Geometry check sheet. Reference: the model listing, model coordinates, mm. A direction names the side the tool comes from. Round coordinates to 2 decimals unless told otherwise and drop trailing zeros. Write each loop counter-clockwise with the first axis right and the second up, starting at its lowest first coordinate (ties: lowest second). Pieces come first, ordered by that corner, then holes. Notation, with made-up numbers: M 20,-26 L 25,-26 A35 cw 25,10 Z; hole C -22.5,72.5 d5. An arc over 180 degrees is marked long. Answer as CSV lines item,"result". Start each with the question number.
```python
from build123d import *

# Parameters (mm, degrees)
F0_W      = 30
F0_H      = 20
F1_DEPTH  = 100
F2_W      = 80
F2_H      = 80
F3_DEPTH  = 60
F4_W      = 10
F4_H      = 10
F5_DEPTH  = 40
F7_DEPTH  = 30
F9_DEPTH  = 30
F10_W     = 10
F10_H     = 10
F11_DEPTH = 30
F12_W     = 40
F12_H     = 85
F13_DEPTH = 25
F15_W     = 33.7672308087
F15_H     = 41.9678427279
F16_DEPTH = 85
F14_W     = 30
F14_H     = 70
F17_DEPTH = 10
F18_W     = 33.7672308087
F18_H     = 41.9678427279
F19_DEPTH = 15
F20_W     = 40.303826414
F20_H     = 30.5195645853
F21_DEPTH = 10
F22_W     = 47.274120152
F22_H     = 29.6948088799
F23_DEPTH = 100
F25_DEPTH = 30
F27_DEPTH = 5


with BuildPart() as f1:
    # F0 (on Top) → F1 (new body)
    with BuildSketch(Plane.XY):
        Polygon((-33.6863899055, 46.2346871942), (-73.6863899055, 46.2346871942), (-73.6863899055, 16.2346871942), (-73.6863899055, -3.7106291857), (-33.6863899055, -3.7653128058), (-33.6863899055, 16.2346871942), align=None)
        Polygon((106.3136100945, 46.2346871942), (-33.6863899055, 46.2346871942), (-33.6863899055, 16.2346871942), (-3.6863899055, 16.2346871942), (106.3136100945, 16.2346871942), align=None)
        with Locations((-18.6863899055, 6.2346871942)):
            Rectangle(F0_W, F0_H)
    extrude(amount=F1_DEPTH)

    # F2 (on face) → F3 (cut)
    with BuildSketch(Plane(origin=(0, 46.2346871942, 0), x_dir=(-1, 0, 0), z_dir=(0, 1, 0))):
        Polygon((-106.3136100945, 100), (-106.3136100945, 0), (-6.3136100945, 100), align=None)
        with Locations((33.6863899055, 40)):
            Rectangle(F2_W, F2_H)
    extrude(amount=-F3_DEPTH, mode=Mode.SUBTRACT)

    # F4 (on face) → F5 (cut)
    with BuildSketch(Plane(origin=(0, 46.2346871942, 0), x_dir=(-1, 0, 0), z_dir=(0, 1, 0))):
        with Locations((-11.3136100945, 95)):
            Rectangle(F4_W, F4_H)
        with Locations((-101.3136100945, 5)):
            Rectangle(F4_W, F4_H)
        with Locations((-91.3136100945, 15)):
            Rectangle(F4_W, F4_H)
        with Locations((-81.3136100945, 25)):
            Rectangle(F4_W, F4_H)
        with Locations((-71.3136100945, 35)):
            Rectangle(F4_W, F4_H)
        with Locations((-61.3136100945, 45)):
            Rectangle(F4_W, F4_H)
        with Locations((-51.3136100945, 55)):
            Rectangle(F4_W, F4_H)
        with Locations((-41.3136100945, 65)):
            Rectangle(F4_W, F4_H)
        with Locations((-31.3136100945, 75)):
            Rectangle(F4_W, F4_H)
        with Locations((-21.3136100945, 85)):
            Rectangle(F4_W, F4_H)
    extrude(amount=-F5_DEPTH, mode=Mode.SUBTRACT)

    # F6 (on face) → F7 (cut)
    with BuildSketch(Plane.YZ.offset(-3.6863899055)):
        Polygon((16.2346871942, 80), (-3.7653128058, 100), (-3.7653128058, 80), align=None)
    extrude(amount=-F7_DEPTH, mode=Mode.SUBTRACT)

    # F8 (on face) → F9 (join)
    with BuildSketch(Plane.YZ.offset(-3.6863899055)):
        Polygon((-3.7653128058, 120), (-3.7653128058, 100), (16.2346871942, 100), align=None)
    extrude(amount=-F9_DEPTH)

    # F10 (on face) → F11 (cut)
    with BuildSketch(Plane.YZ.offset(-3.6863899055)):
        with Locations((11.2346871942, 105)):
            Rectangle(F10_W, F10_H)
        with Locations((1.2346871942, 115)):
            Rectangle(F10_W, F10_H)
    extrude(amount=-F11_DEPTH, mode=Mode.SUBTRACT)

    # F12 (on face) → F13 (join, symmetric)
    with BuildSketch(Plane(origin=(-0.0052104714, -3.8113580263, 0), x_dir=(0.9999990655, -0.0013670892, 0), z_dir=(-0.0013670892, -0.9999990655, 0))):
        with Locations((-53.6812109081, 142.5)):
            Rectangle(F12_W, F12_H)
    extrude(amount=F13_DEPTH, both=True)

    # F15 (on face) → F16 (cut)
    with BuildSketch(Plane.XY.offset(185)):
        with Locations((-53.6770410836, -4.4620987028)):
            Rectangle(F15_W, F15_H)
    extrude(amount=-F16_DEPTH, mode=Mode.SUBTRACT)

    # F14 (on face) → F17 (cut)
    with BuildSketch(Plane(origin=(0.0289667593, 21.188618612, 0), x_dir=(-0.9999990655, 0.0013670892, 0), z_dir=(0.0013670892, 0.9999990655, 0))):
        with Locations((53.6812109081, 135)):
            Rectangle(F14_W, F14_H)
    extrude(amount=-F17_DEPTH, mode=Mode.SUBTRACT)

    # F18 (on face) → F19 (join)
    with BuildSketch(Plane.XY.offset(185)):
        with Locations((-53.6770410836, -4.4620987028)):
            Rectangle(F18_W, F18_H)
    extrude(amount=-F19_DEPTH)

    # F20 (on face) → F21 (join)
    with BuildSketch(Plane(origin=(0, 0, 100), x_dir=(1, 0, 0), z_dir=(0, 0, -1))):
        with Locations((-53.5686165504, 13.4508235825)):
            Rectangle(F20_W, F20_H)
    extrude(amount=F21_DEPTH)

    # F22 (on face) → F23 (cut)
    with BuildSketch(Plane(origin=(0, 0, 90), x_dir=(1, 0, 0), z_dir=(0, 0, -1))):
        with Locations((-54.1594289243, 18.5580336256)):
            Rectangle(F22_W, F22_H)
    extrude(amount=-F23_DEPTH, mode=Mode.SUBTRACT)

    # F24 (on face) → F25 (cut)
    with BuildSketch(Plane(origin=(0, 46.2346871942, 0), x_dir=(-1, 0, 0), z_dir=(0, 1, 0))):
        Polygon((-72.805352509, 0), (-6.3136100945, 0), (-6.3136100945, 80), align=None)
    extrude(amount=-F25_DEPTH, mode=Mode.SUBTRACT)

    # F26 (on face) → F27 (join)
    with BuildSketch(Plane.XZ.offset(-16.2346871942)):
        Polygon((-3.6863899055, 80), (-3.6863899055, 0), (72.805352509, 0), (6.3136100945, 80), align=None)
    extrude(amount=-F27_DEPTH)


solid = f1.part
```
1) Section check C-C, the plane y = 26.5. Record the cut outline in (x, z).
2) Scan lines: line 1 (X direction, y = 0, z = 142); line 2 (Z direction, x = -60.5, y = 17); line 3 (X direction, y = 18, z = 19). Record each from-to range of solid material in increasing order. Write a range as from..to.
3) Access from +Z, -Z, +X, -X, +Y, -Y to the whole of each face (thin tool, end or side, straight path). Record for faces 1 (the flat face through (18, 46.235, 68)), 2 (the flat face through (61, 31, 40)), 3 (the flat face through (26, 21.235, 32)), 4 (the flat face through (-18, 6.235, 105)).
4) Mould release check, pull along X, two halves, no side actions. Record for faces 5 (the flat face through (21, 31, 80)), 6 (the flat face through (46.314, 31, 55)), 7 (the flat face through (-70.561, 6, 135)), 8 (the flat face through (-36.793, 6, 135)): released by +X, released by -X, zero draft, split by the parting line, or undercut.
5) Section check D-D, the plane x = -11. Record the cut outline in (y, z), plus the area to 3 significant figures.
6) Go/stop test with flat-tipped pins: pin 1 (8 mm diameter, centred on y = 10, z = 52.5, fed in from +X) (3 decimals); pin 2 (7 mm diameter, centred on y = 6.5, z = 89.5, fed in from +X); pin 3 (8 mm diameter, centred on x = 91, y = 32, fed in from +Z); pin 4 (3 mm diameter, centred on y = 17.5, z = 117.5, fed in from -X). Record where each tip stops, or that it passes through.
7) Section check A-A, the plane z = 138. Record the cut outline in (x, y), plus the area to 3 significant figures.
Results:
1,outline,"M -73.69,80 L 6.31,80 L 72.81,0 L 96.31,0 L 96.31,10 L 86.31,10 L 86.31,20 L 76.31,20 L 76.31,30 L 66.31,30 L 66.31,40 L 56.31,40 L 56.31,50 L 46.31,50 L 46.31,60 L 36.31,60 L 36.31,70 L 26.31,70 L 26.31,80 L 16.31,80 L 16.31,90 L 6.31,90 L 6.31,100 L -73.69,100 Z"
2,line 1,"x = -73.68..-70.56, -36.79..-33.68"
2,line 2,"z = 80..100, 170..185"
2,line 3,"x = -3.69..86.31"
3,face 1,"+Z, -Z, +X, -X, +Y"
3,face 2,"+Z, +X, +Y, -Y"
3,face 3,"-Z, -X, +Y"
3,face 4,"+Z, +X, +Y"
4,face 5,"zero draft"
4,face 6,"released by +X"
4,face 7,"undercut"
4,face 8,"undercut"
5,outline,"M -3.77,100 L 16.23,80 L 46.23,80 L 46.23,100 L 6.23,100 L 6.23,110 L -3.77,110 Z"
5,area,"900 mm^2"
6,pin 1,"passes through"
6,pin 2,"stops at x = -3.69"
6,pin 3,"stops at z = 10"
6,pin 4,"stops at x = -73.66"
7,outline,"M -73.69,-3.71 L -70.56,-3.71 L -70.56,16.52 L -68.66,16.52 L -68.65,21.28 L -73.65,21.29 Z; M -38.66,16.52 L -36.79,16.52 L -36.79,-3.71 L -33.69,-3.71 L -33.65,21.23 L -38.65,21.24 Z"
7,area,"174 mm^2"
